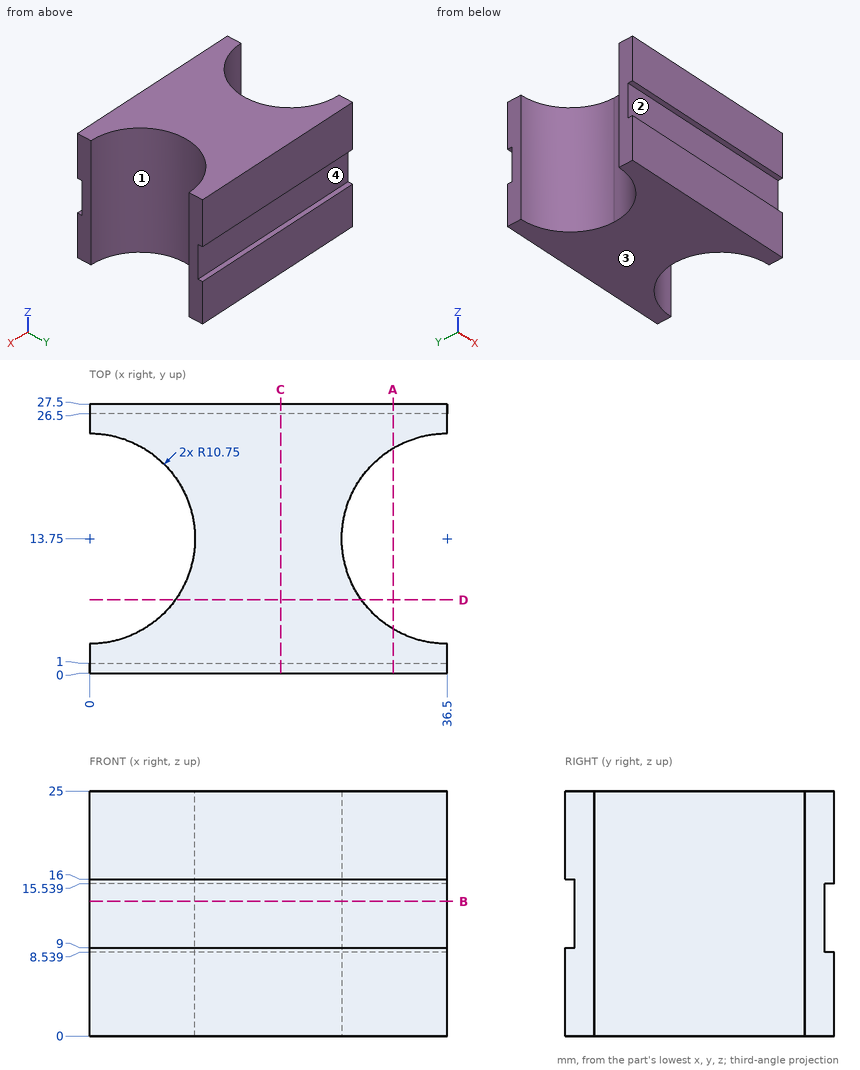
Here's the drawing with two shaded views (mm, measured from the low corner). I have some questions. Round coordinates to 2 decimals unless told otherwise and drop trailing zeros. Loops run counter-clockwise (first coordinate to the right, second up) from the corner with the lowest first, then second, coordinate; pieces in that order, holes last. Notation, with made-up numbers: M 23.25,21 L 54.25,21 A13 cw 54.25,36 Z; hole C 26.25,-31.5 d2. An arc over 180 degrees is marked long. Answer as a JSON object with one key per item and string values. Group by question number.
Q1. We'd pull the mould along Z, two halves only. Please class the marked faces 1, 2, 3 and 4: +Z half, -Z half, draft (parallel to the pull), parting line (faces both ways), or undercut.
Q2. Imagine slicing it at D-D, the plane y = 7.5. Please give me the cut outline in (x, z).
Q3. Please list where these lines run through material, in increasing order: L1, parallel to Y at x = 19, z = 15.5; L2, parallel to Y at x = 34.5, z = 3.75; L3, parallel to X at y = 14, z = 7.75.
Q4. Imagine slicing it at C-C, the plane x = 19.5. Please give me the cut outline in (y, z), then the cut area to 4 significant figures.
Q5. Will these pins go through, and if not, where does the flat tip stop? pin 1 (8 mm diameter, centred on y = 19, z = 16.5, fed in from +X); pin 2 (2 mm diameter, centred on x = 20, z = 13, fed in from -Y); pin 3 (1.5 mm diameter, centred on y = 19, z = 13, fed in from -X).
Q6. Imagine slicing it at B-B, the plane z = 13.75. Please give me the cut outline in (x, y), then the cut area to 3 significant figures.
Q7. Imagine slicing it at A-A, the plane x = 31. Please give me the cut outline in (y, z).
Findings:
{
 "1": {"face 1": "draft", "face 2": "undercut", "face 3": "-Z half", "face 4": "undercut"},
 "2": {"outline": "M 8.75,0 L 27.75,0 L 27.75,25 L 8.75,25 Z"},
 "3": {"L1": "y = 1 to 26.5", "L2": "y = 0 to 3.19, 24.31 to 27.5", "L3": "x = 10.75 to 25.75"},
 "4": {"outline": "M 0,0 L 27.5,0 L 27.5,8.54 L 26.5,8.54 L 26.5,15.54 L 27.5,15.54 L 27.5,25 L 0,25 L 0,16 L 1,16 L 1,9 L 0,9 Z", "area": "673.5 mm2"},
 "5": {"pin 1": "stops at x = 31.02", "pin 2": "stops at y = 1", "pin 3": "stops at x = 8.92"},
 "6": {"outline": "M 0,1 L 36.5,1 L 36.5,3 A10.75 cw 36.5,24.5 L 36.5,26.5 L 0,26.5 L 0,24.5 A10.75 cw 0,3 Z", "area": "568 mm2"},
 "7": {"outline": "M 0,0 L 4.51,0 L 4.51,25 L 0,25 L 0,16 L 1,16 L 1,9 L 0,9 Z; M 22.99,0 L 27.5,0 L 27.5,8.54 L 26.5,8.54 L 26.5,15.54 L 27.5,15.54 L 27.5,25 L 22.99,25 Z"}
}
